Autodesk Inventor part; units mm, degrees
ref_plane "YZ Plane" through (0, 0, 0) normal (1, 0, 0) x (0, 1, 0)
ref_plane "XZ Plane" through (0, 0, 0) normal (0, 1, 0) x (-1, 0, 0)
ref_plane "XY Plane" through (0, 0, 0) normal (0, 0, 1) x (1, 0, 0)
sketch "Sketch1" plane through (0, 0, 0) normal (0, 0, 1) x (1, 0, 0)
  line L0 (-40, -150) -> (70, -150)
  line L1 (70, -150) -> (70, 0)
  line L2 (70, 0) -> (-40, 0)
  line L3 (-40, 0) -> (-40, -30)
  line L4 (-40, -30) -> (0, -30)
  line L5 (0, -30) -> (0, -56)
  line L6 (0, -56) -> (-40, -56)
  line L7 (-40, -56) -> (-40, -67)
  line L8 (-40, -67) -> (0, -67)
  line L9 (0, -67) -> (0, -120)
  line L10 (0, -120) -> (-40, -120)
  line L11 (-40, -120) -> (-40, -150)
  circle A0 centre (-35, -15) radius 2
  circle A1 centre (3.24, -15) radius 2
  line L12 (-35, -15) -> (3.24, -15) construction
  line L13 (-35, -15) -> (-40, -15) construction
  line L14 (-62, 0) -> (92, 0)
  line L15 (0, -180) -> (0, 30)
  circle A2 centre (-35, -61.5) radius 2
  circle A3 centre (3.24, -61.5) radius 2
  line L16 (-35, -61.5) -> (3.24, -61.5) construction
  circle A4 centre (-35, -135) radius 2
  line L17 (-35, -135) -> (3.24, -135) construction
  circle A5 centre (3.24, -135) radius 2
  line L18 (9.12, -7) -> (66.12, -7)
  line L19 (66.12, -7) -> (66.12, -92)
  line L20 (66.12, -92) -> (9.12, -92)
  line L21 (9.12, -92) -> (9.12, -7)
  line L22 (15.62, -99) -> (59.62, -99)
  line L23 (59.62, -99) -> (59.62, -143)
  line L24 (59.62, -143) -> (15.62, -143)
  line L25 (15.62, -143) -> (15.62, -99)
  line L26 (15.62, -99) -> (59.62, -143) construction
  line L27 (15.62, -143) -> (59.62, -99) construction
  circle A6 centre (19.37, -102.75) radius 1.5
  circle A7 centre (19.37, -139.25) radius 1.5
  circle A8 centre (55.87, -139.25) radius 1.5
  circle A9 centre (55.87, -102.75) radius 1.5
  line L28 (19.37, -102.75) -> (19.37, -139.25) construction
  line L29 (19.37, -139.25) -> (55.87, -139.25) construction
  line L30 (55.87, -139.25) -> (55.87, -102.75) construction
  line L31 (55.87, -102.75) -> (19.37, -102.75) construction
  line L32 (37.62, -7) -> (37.62, -92) construction
  line L33 (37.62, -99) -> (37.62, -143) construction
  point P0 (0, 0)
  dimension "d2" = 4
  dimension "d3" = 4
  dimension "d4" = 38.24
  dimension "d5" = 5
  dimension "d6" = 30
  dimension "d7" = 11
  dimension "d8" = 30
  dimension "d11" = 46.5
  dimension "d18" = 46.5
  dimension "d25" = 120
  dimension "d30" = 57
  dimension "d31" = 85
  dimension "d32" = 44
  dimension "d33" = 44
  dimension "d34" = 40
  dimension "d35" = 70
  dimension "d36" = 3
  dimension "d37" = 3
  dimension "d38" = 3
  dimension "d39" = 3
  dimension "d40" = 36.5
  dimension "d42" = 7
  dimension "d43" = 7
  dimension "d44" = 7
  dimension "d45" = 3.88
  dimension "d46" = 3.88
extrude "Extrusion1" add sketch "Sketch1" along normal blind 6 contours L11 L10 L15 L0 | L15 L9 L5 L2 L1 L0 | L8 L7 L6 L15 | L15 L4 L3 L2
sketch "Sketch2" plane through (0, 0, 6) normal (0, 0, 1) x (1, 0, 0)
  line L0 (0, -56) -> (-40, -56)
  line L1 (-40, -56) -> (-40, -67)
  line L2 (-40, -67) -> (0, -67)
  line L3 (0, -67) -> (0, -120)
  line L4 (0, -120) -> (-40, -120)
  line L5 (-40, -120) -> (-40, -150)
  line L6 (-40, -150) -> (70, -150)
  line L7 (70, -150) -> (70, 0)
  line L8 (70, 0) -> (-40, 0)
  line L9 (-40, 0) -> (-40, -30)
  line L10 (-40, -30) -> (0, -30)
  line L11 (0, -30) -> (0, -56)
  circle A0 centre (-35, -15) radius 2
  circle A1 centre (-35, -61.5) radius 2
  circle A2 centre (-35, -135) radius 2
  circle A3 centre (3.24, -15) radius 2
  circle A4 centre (3.24, -61.5) radius 2
  circle A5 centre (3.24, -135) radius 2
  line L12 (15.62, -99) -> (59.62, -99)
  line L13 (59.62, -99) -> (59.62, -143)
  line L14 (59.62, -143) -> (15.62, -143)
  line L15 (15.62, -143) -> (15.62, -99)
  line L16 (9.12, -7) -> (66.12, -7)
  line L17 (66.12, -7) -> (66.12, -92)
  line L18 (66.12, -92) -> (9.12, -92)
  line L19 (9.12, -92) -> (9.12, -7)
  circle A6 centre (19.37, -102.75) radius 1.5
  circle A7 centre (19.37, -139.25) radius 1.5
  circle A8 centre (55.87, -139.25) radius 1.5
  circle A9 centre (55.87, -102.75) radius 1.5
  point P0 (0, 0)
extrude "Extrusion2" add sketch "Sketch2" against normal blind 3 contours L12 L13 L14 L15 | L16 L17 L18 L19
fillet "Fillet1" radius 5 6 edges at (0, -56, 3) (0, -30, 3) (0, -67, 3) (0, -120, 3) (70, 0, 3) (70, -150, 3)
sketch "Sketch3" plane through (0, 0, 6) normal (0, 0, 1) x (1, 0, 0)
  circle A0 centre (-35, -15) radius 2
  circle A1 centre (-35, -15) radius 4
  circle A2 centre (3.24, -15) radius 2
  circle A3 centre (3.24, -15) radius 4
  circle A4 centre (3.24, -61.5) radius 2
  circle A5 centre (3.24, -61.5) radius 4
  circle A6 centre (-35, -61.5) radius 2
  circle A7 centre (-35, -61.5) radius 4
  circle A8 centre (-35, -135) radius 2
  circle A9 centre (-35, -135) radius 4
  circle A10 centre (3.24, -135) radius 2
  circle A11 centre (3.24, -135) radius 4
  circle A12 centre (55.87, -102.75) radius 1.5
  circle A13 centre (55.87, -102.75) radius 3
  circle A14 centre (55.87, -139.25) radius 1.5
  circle A15 centre (55.87, -139.25) radius 3
  circle A16 centre (19.37, -139.25) radius 1.5
  circle A17 centre (19.37, -139.25) radius 3
  circle A18 centre (19.37, -102.75) radius 1.5
  circle A19 centre (19.37, -102.75) radius 3
  point P0 (0, 0)
  dimension "d50" = 8
  dimension "d51" = 8
  dimension "d52" = 8
  dimension "d53" = 8
  dimension "d54" = 8
  dimension "d55" = 8
  dimension "d58" = 6
  dimension "d59" = 6
  dimension "d60" = 6
  dimension "d61" = 6
extrude "Extrusion3" cut sketch "Sketch3" against normal blind 3 contours A0 | A1 | A2 | A3 | A4 | A5 | A6 | A7 | A8 | A9 | A10 | A11
extrude "Extrusion4" cut sketch "Sketch3" against normal blind 2 contours A12 | A13 | A14 | A15 | A16 | A17 | A18 | A19
ref_plane "Work Plane1" through (-0.0065, -108, -32.8761) normal (0, -1, 0) x (-0.1736, 0, -0.9848)
sketch "Sketch5" plane through (-0.0065, -108, -32.8761) normal (0, -1, 0) x (-0.1736, 0, -0.9848)
  line L0 (-20, -17) -> (-20, 0)
  line L1 (-20, 0) -> (-32.9797, -2.2887)
  line L2 (-43.6649, 58.31) -> (-25.4318, -45.0948)
  line L3 (-25.4318, -45.0948) -> (-43.6649, 58.31)
  line L4 (-20, -17) -> (-35.9813, -19.8179)
  line L5 (-37.4183, -11.6684) -> (-31.3406, -46.1367)
  line L6 (-31.3406, -46.1367) -> (-49.5737, 57.2682)
  line L7 (-32.9797, -2.2887) -> (-38.8885, -3.3306)
  line L8 (-38.1546, -7.4928) -> (-39.5438, 0.3857)
  point P0 (-32.3777, -5.7025)
extrude "Extrusion5" add sketch "Sketch5" against normal blind 20
fillet "Fillet2" radius 5 4 edges at (-13.2753, -88, -2.1139) (-13.2753, -108, -2.1139) (0, -88, 3) (0, -108, 3)
equation "\"d11\" = LMaSP"
equation "\"d18\" = LMaSP"
equation "\"d25\" = LM1aM2"
equation "\"d42\" = d44"
equation "\"d43\" = d42"
equation "\"d45\" = d46"
equation "\"d64\" = H1"
equation "\"H1\" = 20"
equation "\"DER\" = 22"
equation "\"HR\" = 7"
equation "\"DIR\" = 8"
equation "\"DEM\" = 4"
equation "\"Dmarc\" = 17.5"
equation "\"Bsm\" = 22.5"
equation "\"Hsm\" = 12"
equation "\"Lsm\" = 21"
equation "\"Dsc\" = 5"
equation "\"RC\" = 7"
equation "\"PB\" = 25"
equation "\"TB\" = 3"
equation "\"HSE\" = 25"
equation "\"LMaSP\" = 46.5"
equation "\"LM1aM2\" = 120"
properties part number "PlacaBase"
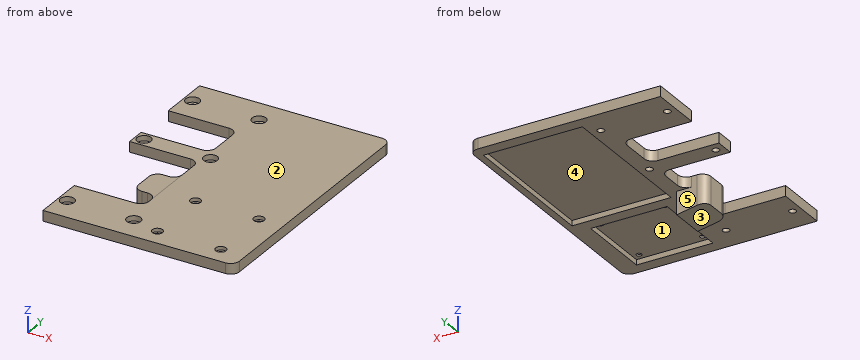
Could you check a few things on this model? Use its own coordinates, in mm. Face numbers are marked on the shaded views. A direction names the side the tool comes from. Coordinates: 2 decimals unless noted, no trailing zeros. Write each loop counter-clockwise with the first axis right and the second up, starting at its lowest first coordinate (ties: lowest second). Pieces come first, ordered by that corner, then holes. Notation, with made-up numbers: M 56,44.25 L 92,44.25 A27 cw 92,68.25 Z; hole C -5.75,-17.75 d7. An arc over 180 degrees is marked long. Answer as CSV lines item,"result". Start each with the question number.
1) For the marked faces 3, 4 and 5, which set-ups out of +Z, -Z, +X, -X, +Y, -Y let a thin tool reach every point of the face, with its end or its side?
2) I want a section at D-D, the plane x = -21.5. Please give me the cut outline in (y, z), and give its area (3 significant figures).
3) I want a section at A-A, the plane x = 55.87. Please give me the cut outline in (y, z), and give its area (3 significant figures).
4) I want a section at C-C, the plane y = -123.5. Please give me the cut outline in (x, z).
5) For P1, Ø5, axis at x = 3.24, y = -61.5, coming from the +Z side; P2, Ø5, axis at x = -35, y = -15, coming from the -Z side; P3, Ø4, axis at x = 55.87, y = -139.25, coming from the +Z side, each with a flat end and sliding along its axis, tell me the tip position at first contact or that it passes through.
6) Please list where these lines run through material, in increasing order: line 1 (X direction, y = -135, z = 1.15); line 2 (Y direction, x = 55.87, z = 4.75); line 3 (Y direction, x = 3.24, z = 4.35). Write a range as from..to.
7) I want a section at B-B, the plane y = -15. Please give me the cut outline in (x, z), and give its area (3 significant figures).
8) We'd pull the mould along Y, two halves only. Please class the marked faces 1 and 2: +Y half, -Y half, draft (parallel to the pull), parting line (faces both ways), or undercut.
Data:
1,face 3,"-Z, -X, +Y, -Y"
1,face 4,"-Z"
1,face 5,"-Z, -X"
2,outline,"M -150,0 L -120,0 L -120,6 L -150,6 Z; M -67,0 L -56,0 L -56,6 L -67,6 Z; M -30,0 L 0,0 L 0,6 L -30,6 Z"
2,area,"426 mm^2"
3,outline,"M -150,0 L -143,0 L -143,3 L -140.75,3 L -140.75,4 L -142.25,4 L -142.25,6 L -150,6 Z; M -137.75,3 L -104.25,3 L -104.25,4 L -105.75,4 L -105.75,6 L -136.25,6 L -136.25,4 L -137.75,4 Z; M -101.25,3 L -99,3 L -99,0 L -92,0 L -92,3 L -7,3 L -7,0 L 0,0 L 0,6 L -99.75,6 L -99.75,4 L -101.25,4 Z"
3,area,"483 mm^2"
4,outline,"M -40,0 L 15.62,0 L 15.62,3 L 59.62,3 L 59.62,0 L 70,0 L 70,6 L -40,6 Z"
5,P1,"stops at z = 3"
5,P2,"stops at z = 0"
5,P3,"stops at z = 4"
6,line 1,"x = -40..-37, -33..1.24, 5.24..15.62, 59.62..70"
6,line 2,"y = -150..-142.25, -136.25..-105.75, -99.75..0"
6,line 3,"y = -150..-139, -131..-65.5, -57.5..-19, -11..0"
7,outline,"M -40,0 L -37,0 L -37,3 L -39,3 L -39,6 L -40,6 Z; M -33,0 L 1.24,0 L 1.24,3 L -0.76,3 L -0.76,6 L -31,6 L -31,3 L -33,3 Z; M 5.24,0 L 9.12,0 L 9.12,3 L 66.12,3 L 66.12,0 L 70,0 L 70,6 L 7.24,6 L 7.24,3 L 5.24,3 Z"
7,area,"417 mm^2"
8,face 1,"undercut"
8,face 2,"draft"
